from build123d import *

# Parameters (mm, degrees)
SKETCH1_W           = 37.9349
SKETCH1_H           = 37.9349
BOSS_EXTRUDE1_DEPTH = 1.651
SKETCH2_W           = 16.002
SKETCH2_H           = 16.002
BOSS_EXTRUDE2_DEPTH = 7.62
SKETCH3_R           = 8.001
BOSS_EXTRUDE3_DEPTH = 6.35
SKETCH4_R           = 5.9309
BOSS_EXTRUDE4_DEPTH = 4.9403
SKETCH5_R           = 6.985
BOSS_EXTRUDE5_DEPTH = 4.2545
SKETCH6_R           = 4.38785
CUT_EXTRUDE1_DEPTH  = 0.635
FILLET2_R           = 2.54
SKETCH9_R           = 1.1176
CUT_EXTRUDE2_DEPTH  = 1.651
SKETCH12_W          = 3.3274
SKETCH12_H          = 4.5466
BOSS_EXTRUDE6_DEPTH = 3.6957
SKETCH13_W          = 10.16
SKETCH13_H          = 4.7117
BOSS_EXTRUDE7_DEPTH = 5.6515
SKETCH14_W          = 4.8006
SKETCH14_H          = 6.0833
BOSS_EXTRUDE8_DEPTH = 5.842
SKETCH15_W          = 3.3528
SKETCH15_H          = 4.5212
BOSS_EXTRUDE9_DEPTH = 4.6101


# Read off the part's stored shape, not the designer's step: Dome1
with BuildPart() as part:
    # Sketch1 → Boss-Extrude1 (new body)
    with BuildSketch(Plane.XY):
        with Locations((18.96745, 18.96745)):
            Rectangle(SKETCH1_W, SKETCH1_H)
    extrude(amount=BOSS_EXTRUDE1_DEPTH)

    # Sketch2 → Boss-Extrude2 (add)
    with BuildSketch(Plane.XY.offset(1.651)):
        with Locations((18.96745, 18.96745)):
            Rectangle(SKETCH2_W, SKETCH2_H)
    extrude(amount=BOSS_EXTRUDE2_DEPTH)

    # Sketch3 → Boss-Extrude3 (add)
    with BuildSketch(Plane.XY.offset(9.271)):
        with Locations((18.96745, 18.96745)):
            Circle(SKETCH3_R)
    extrude(amount=BOSS_EXTRUDE3_DEPTH)

    # Sketch4 → Boss-Extrude4 (add)
    with BuildSketch(Plane.XY.offset(15.621)):
        with Locations((18.96745, 18.96745)):
            Circle(SKETCH4_R)
    extrude(amount=BOSS_EXTRUDE4_DEPTH)

    # Sketch5 → Boss-Extrude5 (add)
    with BuildSketch(Plane.XY.offset(20.5613)):
        with Locations((18.96745, 18.96745)):
            Circle(SKETCH5_R)
    extrude(amount=BOSS_EXTRUDE5_DEPTH)

    # Sketch6 → Cut-Extrude1 (cut)
    with BuildSketch(Plane.XY.offset(24.8158)):
        with Locations((18.96745, 18.96745)):
            Circle(SKETCH6_R)
    extrude(amount=-CUT_EXTRUDE1_DEPTH, mode=Mode.SUBTRACT)

    # Fillet2
    # the kernel refuses this fillet: 2.54 mm, written as the material it takes off along each edge
    with BuildSketch(Plane(origin=(18.96745, 18.96745, 24.8158), x_dir=(1, 0, 0), z_dir=(0, -1, 0))) as fillet2_piece_1:
        with BuildLine():
            CenterArc((6.067902083, -2.54), FILLET2_R, 90, 41.409622109)
            Line((4.38785, -0.635), (4.354248958, -0.5969))
            ThreePointArc((4.354248958, -0.5969), (4.33705, -0.3175), (4.33705, 0))
            Line((4.33705, 0), (4.38785, 0.0508))
            Line((4.38785, 0.0508), (6.067902083, 0.0508))
            Line((6.067902083, 0.0508), (6.067902083, 0))
        make_face()
    revolve(axis=Axis((18.96745, 18.96745, 24.8158), (0, 0, 1)), mode=Mode.SUBTRACT)

    # Dome1 outline → Dome1 (revolve)
    with BuildSketch(Plane(origin=(18.96745, 18.96745, 0), x_dir=(1, 0, 0), z_dir=(0, -1, 0))):
        with BuildLine():
            Line((0, 24.1808), (4.387850012, 24.180799996))
            ThreePointArc((4.387850012, 24.180799996), (2.22676176, 24.75088497), (0, 24.9428))
            Line((0, 24.9428), (0, 24.1808))
        make_face()
    revolve(axis=Axis((18.96745, 18.96745, 0), (0, 0, 1)))

    # Sketch9 → Cut-Extrude2 (cut)
    with BuildSketch(Plane.XY.offset(1.651)):
        with Locations((33.62325, 33.62325)):
            Circle(SKETCH9_R)
        with Locations((4.31165, 33.62325)):
            Circle(SKETCH9_R)
        with Locations((4.31165, 4.31165)):
            Circle(SKETCH9_R)
        with Locations((33.62325, 4.31165)):
            Circle(SKETCH9_R)
        with BuildLine():
            Line((35.385619933, 12.100169933), (35.385619933, 2.549280067))
            Line((35.385619933, 2.549280067), (25.834730067, 2.549280067))
            ThreePointArc((25.834730067, 2.549280067), (25.2984, 2.01295), (25.834730067, 1.476619933))
            Line((25.834730067, 1.476619933), (35.385619933, 1.476619933))
            ThreePointArc((35.385619933, 1.476619933), (37.303202335, 0.631697665), (36.458280067, 2.549280067))
            Line((36.458280067, 2.549280067), (36.458280067, 12.100169933))
            ThreePointArc((36.458280067, 12.100169933), (35.92195, 12.6365), (35.385619933, 12.100169933))
        make_face()
        with BuildLine():
            Line((35.385619933, 36.458280067), (25.834730067, 36.458280067))
            ThreePointArc((25.834730067, 36.458280067), (25.2984, 35.92195), (25.834730067, 35.385619933))
            Line((25.834730067, 35.385619933), (35.385619933, 35.385619933))
            Line((35.385619933, 35.385619933), (35.385619933, 25.834730067))
            ThreePointArc((35.385619933, 25.834730067), (35.92195, 25.2984), (36.458280067, 25.834730067))
            Line((36.458280067, 25.834730067), (36.458280067, 35.385619933))
            ThreePointArc((36.458280067, 35.385619933), (37.303202335, 37.303202335), (35.385619933, 36.458280067))
        make_face()
        with BuildLine():
            Line((12.048880067, 36.458280067), (2.549280067, 36.458280067))
            ThreePointArc((2.549280067, 36.458280067), (0.631697665, 37.303202335), (1.476619933, 35.385619933))
            Line((1.476619933, 35.385619933), (1.476619933, 25.886019933))
            ThreePointArc((1.476619933, 25.886019933), (2.01295, 25.349689867), (2.549280067, 25.886019933))
            Line((2.549280067, 25.886019933), (2.549280067, 35.385619933))
            Line((2.549280067, 35.385619933), (12.048880067, 35.385619933))
            ThreePointArc((12.048880067, 35.385619933), (12.585210133, 35.92195), (12.048880067, 36.458280067))
        make_face()
        with BuildLine():
            Line((23.06955, 36.458280067), (14.86535, 36.458280067))
            ThreePointArc((14.86535, 36.458280067), (14.329019933, 35.92195), (14.86535, 35.385619933))
            Line((14.86535, 35.385619933), (23.06955, 35.385619933))
            ThreePointArc((23.06955, 35.385619933), (23.605880067, 35.92195), (23.06955, 36.458280067))
        make_face()
        with BuildLine():
            Line((2.549280067, 23.06955), (2.549280067, 14.86535))
            ThreePointArc((2.549280067, 14.86535), (2.01295, 14.329019933), (1.476619933, 14.86535))
            Line((1.476619933, 14.86535), (1.476619933, 23.06955))
            ThreePointArc((1.476619933, 23.06955), (2.01295, 23.605880067), (2.549280067, 23.06955))
        make_face()
        with BuildLine():
            Line((36.458280067, 23.06955), (36.458280067, 14.86535))
            ThreePointArc((36.458280067, 14.86535), (35.92195, 14.329019933), (35.385619933, 14.86535))
            Line((35.385619933, 14.86535), (35.385619933, 23.06955))
            ThreePointArc((35.385619933, 23.06955), (35.92195, 23.605880067), (36.458280067, 23.06955))
        make_face()
        with BuildLine():
            Line((23.06955, 2.549280067), (14.86535, 2.549280067))
            ThreePointArc((14.86535, 2.549280067), (14.329019933, 2.01295), (14.86535, 1.476619933))
            Line((14.86535, 1.476619933), (23.06955, 1.476619933))
            ThreePointArc((23.06955, 1.476619933), (23.605880067, 2.01295), (23.06955, 2.549280067))
        make_face()
        with BuildLine():
            Line((2.549280067, 12.100169933), (2.549280067, 2.549280067))
            Line((2.549280067, 2.549280067), (12.100169933, 2.549280067))
            ThreePointArc((12.100169933, 2.549280067), (12.6365, 2.01295), (12.100169933, 1.476619933))
            Line((12.100169933, 1.476619933), (2.600569933, 1.476619933))
            ThreePointArc((2.600569933, 1.476619933), (0.681867267, 0.681867267), (1.476619933, 2.600569933))
            Line((1.476619933, 2.600569933), (1.476619933, 12.100169933))
            ThreePointArc((1.476619933, 12.100169933), (2.01295, 12.6365), (2.549280067, 12.100169933))
        make_face()
    extrude(amount=-CUT_EXTRUDE2_DEPTH, mode=Mode.SUBTRACT)

    # Sketch12 → Boss-Extrude6 (add)
    with BuildSketch(Plane(origin=(0, 0, 0), x_dir=(-1, 0, 0), z_dir=(0, 0, -1))):
        with Locations((-33.721919933, 18.96745)):
            Rectangle(SKETCH12_W, SKETCH12_H)
    extrude(amount=BOSS_EXTRUDE6_DEPTH)

    # Sketch13 → Boss-Extrude7 (add)
    with BuildSketch(Plane(origin=(0, 0, 0), x_dir=(-1, 0, 0), z_dir=(0, 0, -1))):
        with Locations((-23.8125, 4.905130067)):
            Rectangle(SKETCH13_W, SKETCH13_H)
    extrude(amount=BOSS_EXTRUDE7_DEPTH)

    # Sketch14 → Boss-Extrude8 (add)
    with BuildSketch(Plane(origin=(0, 0, 0), x_dir=(-1, 0, 0), z_dir=(0, 0, -1))):
        with Locations((-4.949580067, 12.02055)):
            Rectangle(SKETCH14_W, SKETCH14_H)
    extrude(amount=BOSS_EXTRUDE8_DEPTH)

    # Sketch15 → Boss-Extrude9 (add)
    with BuildSketch(Plane(origin=(0, 0, 0), x_dir=(-1, 0, 0), z_dir=(0, 0, -1))):
        with Locations((-4.225680067, 17.3228)):
            Rectangle(SKETCH15_W, SKETCH15_H)
    extrude(amount=BOSS_EXTRUDE9_DEPTH)


solid = part.part
Model file for the job. Use its own axes, mm. A direction names the side the tool comes from. Give positions to 0.01 mm unless a question says otherwise; leave off trailing zeros. Loops run counter-clockwise (first coordinate to the right, second up) from the corner with the lowest first, then second, coordinate; pieces in that order, holes last.
Item 1: Slice it at D-D (x = 22.5). Give the number of separate pieces and of enclosed holes in the cut face, plus the area to 3 significant figures.
Check values:
separate pieces: 3
enclosed holes: 0
area: 394 mm2
Item 2: Drop flat-ended pins along their axis: P1, Ø10, axis at x = 20.5, y = 8, coming from the -Z side; P2, Ø6.5, axis at x = 23, y = 14, coming from the +Z side; P3, Ø1.5, axis at y = 18.5, z = 11, coming from the +X side; P4, Ø1.3, axis at x = 1.43, y = 36.51, coming from the +Z side. Give the stop position or say it passes through.
Check values:
P1: stops at z = -5.65
P2: stops at z = 24.82
P3: stops at x = 26.97
P4: passes through
Item 3: Slice it at C-C (z = 4.5). Write the cut outline in (x, y), plus the area to 3 significant figures.
Check values:
outline: (10.97, 10.97) - (26.97, 10.97) - (26.97, 26.97) - (10.97, 26.97) - close
area: 256 mm2
Item 4: Mould opens along Y. For faces 4 (the face through (19, 36.458, 1)), 5 (the face through (4, 19.583, -2)), 6 (the face through (13.6, 16, 15.621)) say: +Y half, -Y half, draft (parallel to the pull), parting line (faces both ways), or undercut.
Check values:
face 4: undercut
face 5: +Y half
face 6: draft
Item 5: Drill centre lines: line 1 along X through (y, z) = (17.5, 0.5); line 2 along Y through (x, z) = (33.5, 1); line 3 along X through (y, z) = (26, 8). Where is each one in solid material? Low to high.
Check values:
line 1: x = 0 to 1.48, 2.55 to 35.39, 36.46 to 37.93
line 2: y = 0 to 1.48, 2.55 to 3.2, 5.42 to 32.51, 34.73 to 35.39, 36.46 to 37.93
line 3: x = 10.97 to 26.97
Item 6: Slice it at A-A (y = 8). Write the cut outline in (x, z).
Check values:
outline: (0, 0) - (1.48, 0) - (1.48, 1.65) - (0, 1.65) - close; (2.55, 0) - (35.39, 0) - (35.39, 1.65) - (2.55, 1.65) - close; (36.46, 0) - (37.93, 0) - (37.93, 1.65) - (36.46, 1.65) - close
Item 7: Which spindle directions (+Z, -Z, +X, -X, +Y, -Y) get a long thin tool onto all of the face, cutting with end or side? Do faces 1 (the face through (35.386, 31, 1)), 2 (the face through (24, 7.261, -3)), 3 (the face through (13, 13, 9.271)). Say none if no direction does.
Check values:
face 1: +Z, -Z
face 2: -Z, +X, -X, +Y
face 3: +Z, -X, -Y
Item 8: Slice it at B-B (x = 4). Write the cut outline in (y, z).
Check values:
outline: (0, 0) - (1.48, 0) - (1.48, 1.65) - (0, 1.65) - close; (2.55, 0) - (3.24, 0) - (3.24, 1.65) - (2.55, 1.65) - close; (5.38, 0) - (8.98, 0) - (8.98, -5.84) - (15.06, -5.84) - (15.06, -4.61) - (19.58, -4.61) - (19.58, 0) - (32.55, 0) - (32.55, 1.65) - (5.38, 1.65) - close; (34.7, 0) - (35.39, 0) - (35.39, 1.65) - (34.7, 1.65) - close; (36.46, 0) - (37.93, 0) - (37.93, 1.65) - (36.46, 1.65) - close
